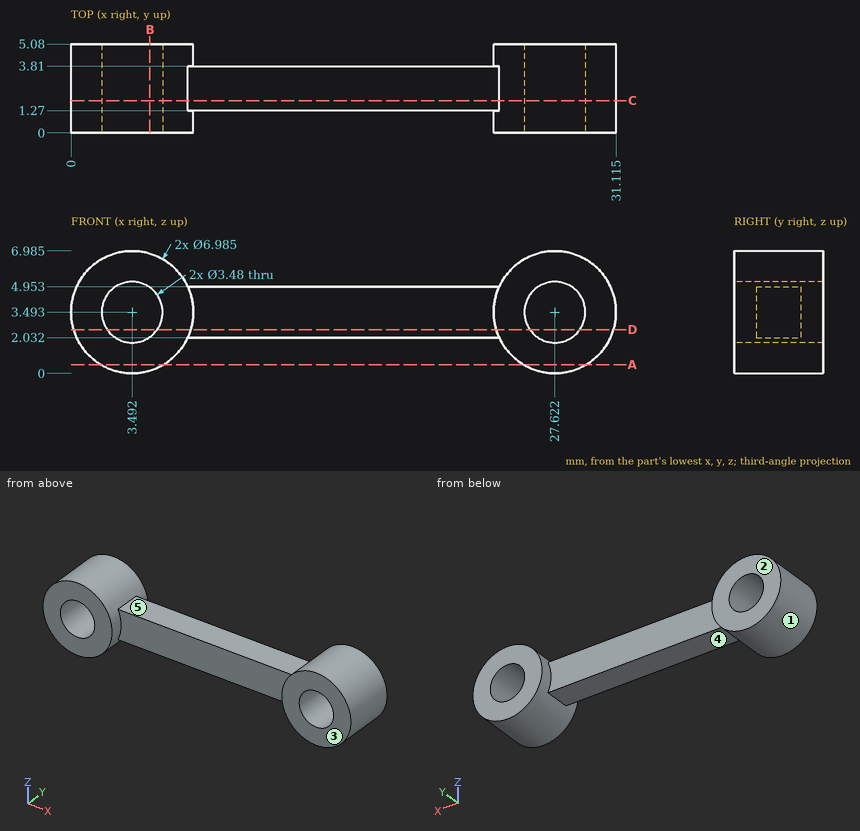
Verification items for this drawing (mm, ordinates from the low corner). A direction names the side the tool comes from. Round coordinates to 2 decimals unless told otherwise and drop trailing zeros. Loops run counter-clockwise (first coordinate to the right, second up) from the corner with the lowest first, then second, coordinate; pieces in that order, holes last. Notation, with made-up numbers: M -1,75.5 L 32,75.5 A14 cw 32,84.5 Z; hole C 65.25,6 d2. An arc over 180 degrees is marked long. Answer as a JSON object with one key per item and string values.
1. Section check A-A (z = 0.5). Record the boundary of the cut face in (x, y), plus the area to 3 significant figures.
Reply:
{"outline": "M 1.69,0 L 5.29,0 L 5.29,5.08 L 1.69,5.08 Z; M 25.82,0 L 29.42,0 L 29.42,5.08 L 25.82,5.08 Z", "area": "36.6 mm²"}
2. Access from +Z, -Z, +X, -X, +Y, -Y to the whole of each face (thin tool, end or side, straight path). Record for the marked faces 3, 4 and 5.
Reply:
{"face 3": "+Z, -Z, +X, -X, -Y", "face 4": "-Z, +Y, -Y", "face 5": "+Z, +Y, -Y"}
3. Section check B-B (x = 4.5). Record the boundary of the cut face in (y, z).
Reply:
{"outline": "M 0,0.15 L 5.08,0.15 L 5.08,2.07 L 0,2.07 Z; M 0,4.91 L 5.08,4.91 L 5.08,6.84 L 0,6.84 Z"}
4. Section check D-D (z = 2.5). Record the boundary of the cut face in (x, y) (1 decimal).
Reply:
{"outline": "M 0.1,0 L 2.1,0 L 2.1,5.1 L 0.1,5.1 Z; M 4.9,0 L 6.8,0 L 6.8,1.3 L 24.3,1.3 L 24.3,0 L 26.2,0 L 26.2,5.1 L 24.3,5.1 L 24.3,3.8 L 6.8,3.8 L 6.8,5.1 L 4.9,5.1 Z; M 29.1,0 L 31,0 L 31,5.1 L 29.1,5.1 Z"}
5. Mould release check, pull along X, two halves, no side actions. Record for the marked faces 1 and 2: pulls with the +X half, pulls with the -X half, needs draft (parallel to the pull), parting line crosses it, or undercut.
Reply:
{"face 1": "undercut", "face 2": "needs draft"}
6. Gauge pin test, flat ends, axial feed: P1, Ø2, axis at y = 2.5, z = 3, coming from the -X side; P2, Ø1.5, axis at x = 12, y = 1.5, coming from the -Z side; P3, Ø1.5, axis at x = 12.5, z = 3, coming from the -Y side; P4, Ø2, axis at y = 3, z = 5, coming from the +X side. Record the tip position at first contact, or that the pin passes through.
Reply:
{"P1": "stops at x = 0", "P2": "stops at z = 2.03", "P3": "stops at y = 1.27", "P4": "stops at x = 31.08"}
7. Scan lines: line 1 (X direction, y = 4.75, z = 3.5) (1 decimal); line 2 (X direction, y = 2.75, z = 3) (1 decimal); line 3 (X direction, y = 4.55, z = 3.75) (1 decimal). Record each from-to range of solid material in increasing order.
Reply:
{"line 1": "x = 0 to 1.8, 5.2 to 7, 24.1 to 25.9, 29.4 to 31.1", "line 2": "x = 0 to 1.8, 5.2 to 26, 29.3 to 31.1", "line 3": "x = 0 to 1.8, 5.2 to 7, 24.1 to 25.9, 29.3 to 31.1"}
8. Section check C-C (y = 1.85). State how many separate pieces and enclosed holes the cut face has, plus the area to 3 significant figures.
Reply:
{"separate pieces": "1", "enclosed holes": "2", "area": "108 mm²"}
